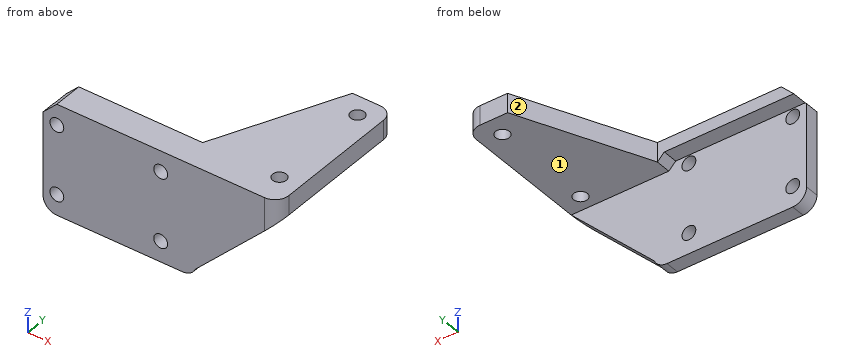
Autodesk Inventor part; units mm, degrees
ref_plane "YZ Plane" through (0, 0, 0) normal (1, 0, 0) x (0, 1, 0)
ref_plane "XZ Plane" through (0, 0, 0) normal (0, 1, 0) x (-1, 0, 0)
ref_plane "XY Plane" through (0, 0, 0) normal (0, 0, 1) x (1, 0, 0)
sketch "Sketch1" plane through (0, 0, 0) normal (0, 0, 1) x (1, 0, 0)
  line L0 (22.5, 10) -> (28.5, 10)
  line L1 (28.5, 10) -> (28.5, -10)
  line L2 (28.5, -10) -> (22.5, -10)
  line L3 (22.5, -10) -> (22.5, 10)
  line L4 (22.5, -10) -> (-28.5, -10)
  line L5 (-28.5, -10) -> (-28.5, -8)
  line L6 (-28.5, -8) -> (22.5, -8)
  line L7 (22.5, -8) -> (22.5, -10)
  circle A0 centre (25.5, 7) radius 1
  circle A1 centre (25.5, -8) radius 1
  point P0 (0, 0)
  dimension "d0" = 57
  dimension "d1" = 2
  dimension "d2" = 28.5
  dimension "d3" = 20
  dimension "d4" = 10
  dimension "d5" = 54
  dimension "d6" = 54
  dimension "d7" = 2
  dimension "d8" = 17
  dimension "d9" = 3
  dimension "d10" = 3
  dimension "d11" = 2
  dimension "d12" = 2
extrude "Extrusion1" add sketch "Sketch1" along normal blind 3
sketch "Sketch2" plane through (0, 0, 3) normal (0, 0, 1) x (1, 0, 0)
  line L0 (-28.5, -10) -> (28.5, -10)
  line L1 (28.5, 10) -> (22.5, 10)
  line L2 (13.5, -10) -> (22.5, 10)
  line L3 (22.5, -8) -> (-28.5, -8)
  line L4 (22.5, 10) -> (22.5, -8)
  line L5 (22.5, -8) -> (13.5, -10)
  point P0 (0, 0)
  point P1 (14.4, -8)
  dimension "d15" = 42
extrude "Extrusion2" add sketch "Sketch2" against normal blind 3 contours L2 L4 L3
sketch "Sketch4" plane through (-28.5, -10, 0) normal (0, -1, 0) x (1, 0, 0)
  line L0 (0, 3) -> (57, 3)
  line L1 (0, 3) -> (57, 3)
  line L2 (57, 3) -> (57, -13)
  line L3 (57, -13) -> (0, -13)
  line L4 (0, -13) -> (0, 3)
  line L5 (57, 0) -> (57, 3)
  point P0 (28.5, 0)
  dimension "d22" = 16
extrude "Extrusion4" add sketch "Sketch4" along normal blind 2.2
sketch "Sketch5" plane through (-28.5, -10, 0) normal (0, 1, 0) x (1, 0, 0)
  line L0 (0, 0) -> (57, 0)
  line L1 (0, 13) -> (57, 13)
  line L2 (0, 0) -> (57, 0)
  line L3 (57, 0) -> (57, 13)
  line L4 (57, 13) -> (0, 13)
  line L5 (0, 13) -> (0, 0)
  point P0 (28.5, 0)
extrude "Extrusion5" cut sketch "Sketch5" against normal blind 0.2
sketch "Sketch6" plane through (0, 0, 0) normal (0, 0, -1) x (-1, 0, 0)
  line L0 (-28.5, 10) -> (-28.5, -12.2)
  line L1 (-28.5, -10.2) -> (28.5, -10.2)
  line L2 (-28.5, 10) -> (28.5, 10)
  line L3 (28.5, 10) -> (28.5, -10.2)
  line L4 (28.5, -10.2) -> (-28.5, -10.2)
  line L5 (-28.5, -10.2) -> (-28.5, 10)
  point P0 (0, 0)
extrude "Extrusion6" cut sketch "Sketch6" against normal blind 0.2
sketch "Sketch7" plane through (-28.5, -12.2, 0) normal (0, -1, 0) x (1, 0, 0)
  line L0 (0, 3) -> (0, -13)
  line L1 (57, 3) -> (0, 3)
  point P0 (28.5, 0)
  point P1 (25, 0)
  point P2 (25, -10)
  point P3 (40, 0)
  point P4 (40, -10)
  dimension "d29" = 25
  dimension "d30" = 40
  dimension "d31" = 25
  dimension "d32" = 40
  dimension "d33" = 10
  dimension "d34" = 10
  dimension "d35" = 3
  dimension "d36" = 3
hole "Hole1" at (-3.5, -12.2, 0) at (-3.5, -12.2, -10) at (11.5, -12.2, 0) at (11.5, -12.2, -10) direction (0, 1, 0) diameter 2 depth 5 tip angle 118
sketch "Sketch8" plane through (-28.5, -8, 3) normal (0, 1, 0) x (1, 0, 0)
  line L0 (42.9, 2.8) -> (40.9798, 2.8)
  line L1 (42.9, 2.8) -> (20.9, 2.8)
  line L2 (20.9, 2.8) -> (20.9, 1.8)
  line L3 (20.9, 1.8) -> (42.9, 1.8)
  line L4 (42.9, 1.8) -> (42.9, 2.8)
  point P0 (28.5, 3)
  dimension "d44" = 22
  dimension "d45" = 1
extrude "Extrusion7" cut sketch "Sketch8" against normal blind 2.2
chamfer "Chamfer1" distance 1 angle 45 2 edges at (-7.6, -9.1, 0.2) (14.4, -9.1, 1.2)
sketch "Sketch9" plane through (-28.5, -12.2, 0) normal (0, -1, 0) x (1, 0, 0)
  line L0 (0, 3) -> (0, -13)
  line L1 (0, -13) -> (57, -13)
  line L2 (0, 3) -> (23, 3)
  line L3 (23, 3) -> (23, -13)
  line L4 (23, -13) -> (0, -13)
  line L5 (0, -13) -> (0, 3)
  point P0 (28.5, 0)
  dimension "d51" = 23
extrude "Extrusion8" cut sketch "Sketch9" against normal blind 5
chamfer "Chamfer2" distance 2 angle 45 1 edges at (-5.5, -10.1, 3)
sketch "Sketch10" plane through (-28.5, -10.2, 0) normal (0, 1, 0) x (1, 0, 0)
  line L0 (57, -0.2) -> (51, -0.2)
  line L1 (23, 13) -> (57, 13)
  line L2 (57, -0.2) -> (45, -0.2)
  line L3 (45, -0.2) -> (45, 13)
  line L4 (45, 13) -> (57, 13)
  line L5 (57, 13) -> (57, -0.2)
  circle A0 centre (40, 0) radius 1
  point P0 (28.5, 0)
  dimension "d57" = 5
extrude "Extrusion9" cut sketch "Sketch10" against normal blind 3 contours L0 L2 L3 L1 L5
chamfer "Chamfer3" distance 12 angle 45 1 edges at (16.5, -11.2, 0.2)
fillet "Fillet2" radius 2 2 edges at (16.5, -11.2, -13) (-5.5, -11.2, -13)
fillet "Fillet3" radius 2 2 edges at (28.5, 10, 1.6) (28.5, -12.2, 1.6)
properties part number "bridge_structure_B"
Model file for the job. Use its own axes, mm. Face numbers are marked on the shaded views. A direction names the side the tool comes from. Coordinates: 2 decimals unless noted, no trailing zeros. Loops run counter-clockwise (first coordinate to the right, second up) from the corner with the lowest first, then second, coordinate; pieces in that order, holes last. Notation, with made-up numbers: (-36.5, 47.5) -> (5.5, 47.5) arc R29 cw to (5.5, 81.5) -> close; hole circle Ø9 at (8.25, 77). An arc over 180 degrees is marked (long way). Answer as a JSON object with one key per item and string values.
Q1. Cut at A-A (x = 11.5). List the corners of the cut face in (y, z), and give its area (3 significant figures).
Report:
{"outline": "(-12.2, -13) -> (-10.2, -13) -> (-10.2, -11) -> (-12.2, -11) -> close; (-12.2, -9) -> (-10.2, -9) -> (-10.2, -1) -> (-12.2, -1) -> close; (-12.2, 1) -> (-10.2, 1) -> (-10.2, 1.2) -> (-8, 1.2) -> (-8, 3) -> (-12.2, 3) -> close", "area": "28.0 mm2"}
Q2. 3-axis set-ups, long thin cutter, end or side, ignore diameter. For the marked faces 1 and 2: which of +Z, -Z, +X, -X, +Y, -Y reach the whole face in a straight line?
Report:
{"face 1": "-Z, +X, -X, +Y", "face 2": "+Z, -Z, -X, +Y"}
Q3. Probe probe 1 along Z at (x, y) = (-3.5, -10.65); probe 2 along Y at (x, z) = (25.5, 1.65); probe 3 along X at (y, z) = (-11.5, 0). List the from-to ranges inside material, lowest first.
Report:
{"probe 1": "z = -13 to -11, -9 to -1, 1 to 3", "probe 2": "y = -12.2 to -9, -7 to 6, 8 to 10", "probe 3": "x = -5.5 to -4.5, -2.5 to 10.5, 12.5 to 28.02"}
Q4. Cut at B-B (z = -10). List the corners of the cut face in (x, y).
Report:
{"outline": "(-5.5, -12.2) -> (-4.5, -12.2) -> (-4.5, -10.2) -> (-5.5, -10.2) -> close; (-2.5, -12.2) -> (10.5, -12.2) -> (10.5, -10.2) -> (-2.5, -10.2) -> close; (12.5, -12.2) -> (18.3, -12.2) -> (18.3, -10.2) -> (12.5, -10.2) -> close"}
Q5. Cut at D-D (x = 25.5). List the corners of the cut face in (y, z).
Report:
{"outline": "(-12.2, -2.8) -> (-10.2, -2.8) -> (-10.2, 0.2) -> (-9, 0.2) -> (-9, 3) -> (-12.2, 3) -> close; (-7, 0.2) -> (6, 0.2) -> (6, 3) -> (-7, 3) -> close; (8, 0.2) -> (10, 0.2) -> (10, 3) -> (8, 3) -> close"}
Q6. Flat gauge pins, fed straight in: P1, Ø1.6, axis at x = 25.5, y = 7, coming from the -Z side; P2, Ø8, axis at x = -0.5, z = -5, coming from the +Y side; P3, Ø5, axis at y = -4.5, z = 1, coming from the -X side; P4, Ø1.4, axis at x = 4, z = 2, coming from the +Y side. Where does each tip first touch, or does it go through?
Report:
{"P1": "passes through", "P2": "stops at y = -10.2", "P3": "stops at x = 14.85", "P4": "stops at y = -8"}
Q7. Cut at C-C (y = -1). List the corners of the cut face in (x, z), and give its area (3 significant figures).
Report:
{"outline": "(17.55, 0.2) -> (28.5, 0.2) -> (28.5, 3) -> (17.55, 3) -> close", "area": "30.7 mm2"}
